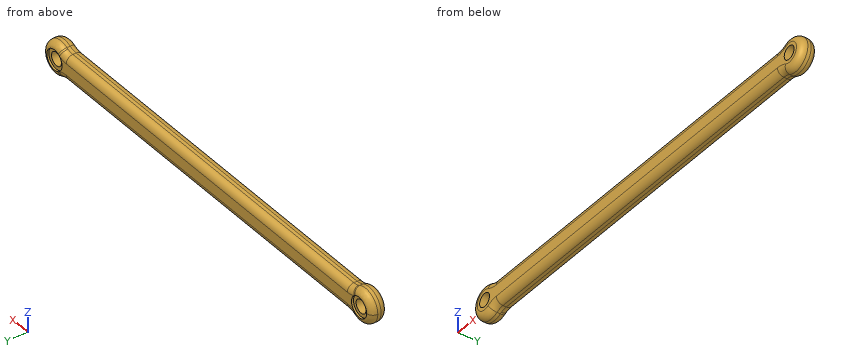
from build123d import *

# Parameters (mm, degrees)
SALIENTE_EXTRUIR1_DEPTH                              = 5
REFRENTADO_PARA_TORNILLO_CON_CABEZA_PLAN_D           = 8.1
REFRENTADO_PARA_TORNILLO_CON_CABEZA_PLAN_CBORE_D     = 12.4
REFRENTADO_PARA_TORNILLO_CON_CABEZA_PLAN_CBORE_DEPTH = 1.2
REDONDEO7_R                                          = 10
REDONDEO6_R                                          = 4


with BuildPart() as part:
    # Croquis1 → Saliente-Extruir1 (new, symmetric)
    with BuildSketch(Plane(origin=(0, 0, 0), x_dir=(-1, 0, 0), z_dir=(0, 1, 0))):
        with BuildLine():
            Line((6.614378278, -7.5), (243.385621722, -7.5))
            ThreePointArc((243.385621722, -7.5), (260, 0), (243.385621722, 7.5))
            Line((243.385621722, 7.5), (6.614378278, 7.5))
            ThreePointArc((6.614378278, 7.5), (-10, 0), (6.614378278, -7.5))
        make_face()
    extrude(amount=SALIENTE_EXTRUIR1_DEPTH, both=True)

    # Refrentado para tornillo con cabeza plana de M81 (through all)
    with Locations(Plane(origin=(0, 5, 0), x_dir=(-1, 0, 0), z_dir=(0, 1, 0))):
        with Locations((0, 0), (250, 0)):
            CounterBoreHole(REFRENTADO_PARA_TORNILLO_CON_CABEZA_PLAN_D / 2, REFRENTADO_PARA_TORNILLO_CON_CABEZA_PLAN_CBORE_D / 2, REFRENTADO_PARA_TORNILLO_CON_CABEZA_PLAN_CBORE_DEPTH)

    # Redondeo7
    redondeo7_edges = [part.edges().sort_by_distance(p)[0] for p in [
        (-243.385621722, 0, -7.5),
        (-6.614378278, 0, -7.5),
        (-6.614378278, 0, 7.5),
        (-243.385621722, 0, 7.5),
    ]]
    fillet(redondeo7_edges, radius=REDONDEO7_R)

    # Redondeo6
    redondeo6_edges = [part.edges().sort_by_distance(p)[0] for p in [
        (-260, -5, 0),
        (-125, 5, 7.5),
        (-125, -5, 7.5),
        (-125, 5, -7.5),
        (-125, -5, -7.5),
        (-7.182458366, -5, -7.817541634),
        (-7.182458366, -5, 7.817541634),
        (-242.817541634, -5, 7.817541634),
        (-242.817541634, -5, -7.817541634),
        (-7.182458366, 5, -7.817541634),
        (-7.182458366, 5, 7.817541634),
        (-242.817541634, 5, 7.817541634),
        (-242.817541634, 5, -7.817541634),
        (10, -5, 0),
    ]]
    fillet(redondeo6_edges, radius=REDONDEO6_R)


solid = part.part
Part model, mm, in its own coordinate system. Give positions to 0.01 mm unless a question says otherwise; leave off trailing zeros. Order: outer loops, then holes, each group sorted by start corner. A loop starts at its lowest first (then second) coordinate and runs counter-clockwise, first axis right, second up. Notation, with made-up numbers: (52, 18) - (106, 18) arc R27 cw to (106, 44) - close; hole circle Ø7 at (-8, 4). An arc over 180 degrees is marked (long way). Use a Markdown table: item, result.
1) Flat gauge pins, fed straight in: P1, Ø4, axis at y = -3, z = -4.5, coming from the +X side; P2, Ø1, axis at x = -231.5, z = -4.5, coming from the +Y side; P3, Ø1.5, axis at x = -222, y = -1.5, coming from the +Z side. Where does each tip first touch, or does it go through?
Checked values:
| item | result |
|---|---|
| P1 | x = 9.49 |
| P2 | y = 4.97 |
| P3 | z = 7.5 |
2) Saw through at B-B on y = -2.75. List the corners of the cut face in (x, z).
Checked values:
| item | result |
|---|---|
| outline | (-245.35, -8.4) arc R10.4 cw to (-240.32, -7.1) - (-9.68, -7.1) arc R10.4 cw to (-4.65, -8.4) arc R9.6 ccw (long way) to (-4.65, 8.4) arc R10.4 cw to (-9.68, 7.1) - (-240.32, 7.1) arc R10.4 cw to (-245.35, 8.4) arc R9.6 ccw (long way) to start; hole circle Ø8.1 at (-250, 0); hole circle Ø8.1 at (0, 0) |
3) Probe L1, parallel to X at y = -1, z = 0.5; L2, parallel to X at y = -3, z = 1.75; L3, parallel to Y at x = -226.5, z = -5. List the from-to ranges inside material, lowest first. Write a range as from..to.
Checked values:
| item | result |
|---|---|
| L1 | -259.99..-254.02, -245.98..-4.02, 4.02..9.99 |
| L2 | -259.3..-253.65, -246.35..-3.65, 3.65..9.3 |
| L3 | -4.71..4.71 |
4) Saw through at A-A on x = -138. List the corners of the cut face in (y, z).
Checked values:
| item | result |
|---|---|
| outline | (-5, -3.5) arc R4 ccw to (-1, -7.5) - (1, -7.5) arc R4 ccw to (5, -3.5) - (5, 3.5) arc R4 ccw to (1, 7.5) - (-1, 7.5) arc R4 ccw to (-5, 3.5) - close |
